Drawing for the job (mm, zero at the part's lowest x, y, z). Round coordinates to 2 decimals unless told otherwise and drop trailing zeros. Order: outer loops, then holes, each group sorted by start corner. A loop starts at its lowest first (then second) coordinate and runs counter-clockwise, first axis right, second up. Notation, with made-up numbers: (47.5, 75.5) -> (79.5, 75.5) arc R30 ccw to (79.5, 114.5) -> close; hole circle Ø1 at (-16, 8). An arc over 180 degrees is marked (long way). Use CSV: the item, a comma, the result in double quotes.
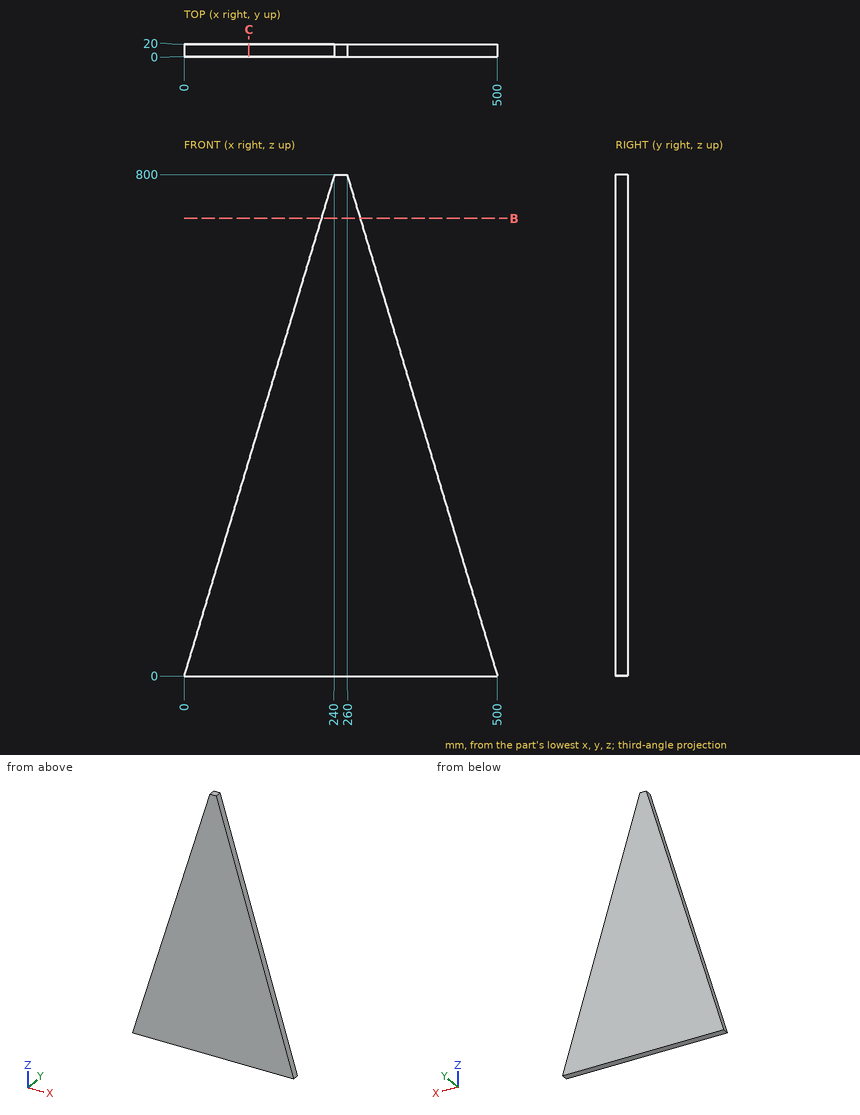
Q1. Cut at B-B (z = 730). Give the cut face in (x, y), plus the area to 3 significant figures.
From the geometry:
outline,"(219, 0) -> (281, 0) -> (281, 20) -> (219, 20) -> close"
area,"1,240 mm²"
Q2. Cut at C-C (x = 103.5). Give the cut face in (y, z).
From the geometry:
outline,"(0, 0) -> (20, 0) -> (20, 345) -> (0, 345) -> close"
Q3. Probe line 1 along X through (y, z) = (17.75, 711.5); line 2 along X through (y, z) = (3.25, 399). List the from-to ranges inside material, lowest first.
From the geometry:
line 1,"x = 213.45 to 286.55"
line 2,"x = 119.7 to 380.3"
Q4. Pin check, flat tips, straight feed: pin 1 (12 mm diameter, centred on y = 11.5, z = 274.5, fed in from +X); pin 2 (4 mm diameter, centred on y = 2, z = 369.5, fed in from -X); pin 3 (10 mm diameter, centred on y = 8, z = 462, fed in from -X). Stop position of each tip, or through.
From the geometry:
pin 1,"stops at x = 419.45"
pin 2,"stops at x = 110.25"
pin 3,"stops at x = 137.1"
